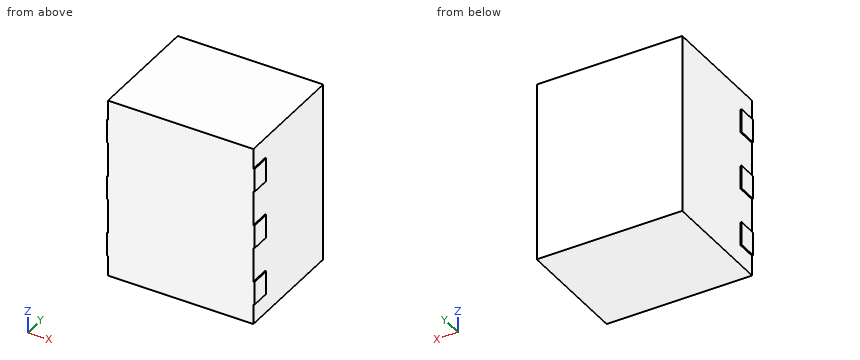
Autodesk Inventor part; units mm, degrees
ref_plane "YZ Plane" through (0, 0, 0) normal (1, 0, 0) x (0, 1, 0)
ref_plane "XZ Plane" through (0, 0, 0) normal (0, 1, 0) x (-1, 0, 0)
ref_plane "XY Plane" through (0, 0, 0) normal (0, 0, 1) x (1, 0, 0)
sketch "Sketch1" plane through (0, 0, 0) normal (0, 1, 0) x (-1, 0, 0)
  line L0 (3.175, 3.935) -> (-3.175, 3.935)
  line L1 (-3.175, 3.935) -> (-3.175, -3.935)
  line L2 (-3.175, -3.935) -> (3.175, -3.935)
  line L3 (3.175, -3.935) -> (3.175, 3.935)
  point P0 (0, 0)
  dimension "d0" = 6.35
  dimension "d1" = 3.175
  dimension "d2" = 7.87
  dimension "d3" = 3.935
extrude "Extrusion1" add sketch "Sketch1" along normal blind 5.08
sketch "Sketch2" plane through (0, 0, 0) normal (0, -1, 0) x (1, 0, 0)
  line L0 (3.225, 0.51) -> (1.955, 0.51)
  line L1 (1.955, 0.51) -> (1.955, -0.51)
  line L2 (1.955, -0.51) -> (3.225, -0.51)
  line L3 (3.225, -0.51) -> (3.225, 0.51)
  line L4 (3.175, 3.935) -> (3.175, -3.935)
  point P0 (0, 0)
  dimension "d6" = 1.02
  dimension "d7" = 0.51
  dimension "d8" = 0.05
  dimension "d9" = 1.27
extrude "Extrusion2" add sketch "Sketch2" against normal blind 0.8467
pattern_linear "Rectangular Pattern1" count 3 spacing 2.54 along (0, 0, -1) of "Extrusion2" first direction both ways yes
mirror "Mirror1" about plane through (0, 0, 0) normal (1, 0, 0) of "Extrusion2", "Rectangular Pattern1"
properties part number "MC_TT240"
The model under review builds one solid part; all positions refer to its coordinate system, in mm. Coordinates: 2 decimals unless noted, no trailing zeros. Order: outer loops, then holes, each group sorted by start corner. A loop starts at its lowest first (then second) coordinate and runs counter-clockwise, first axis right, second up. Notation, with made-up numbers: (-9.75, -22.5) -> (25.25, -22.5) arc R24 cw to (25.25, 0.5) -> close; hole circle Ø8 at (28, 75). An arc over 180 degrees is marked (long way). Answer in a Markdown table with one row per item. Add a question column.
Item 1: Clearance check with a flat-ended pin moving along its axis: pin 1 (1 mm diameter, centred on y = 4.5, z = 3, fed in from -X) (3 decimals). State where the tip first meets the part, or that it passes through.
Item 2: We need section A-A on y = 2.6. Write out the cut boundary in (x, z) (3 decimals).
Item 3: To check wall thickness, follow probe 1 along X at (y, z) = (4.85, -1.5) (3 decimals). State the ranges of the line that lie inside material, in increasing order.
Item 4: We need section B-B on z = 1.5. Write out the cut boundary in (x, y) (3 decimals), plus the area to 3 significant figures.
Final values:
| question | item | result |
|---|---|---|
| 1 | pin 1 | stops at x = -3.175 |
| 2 | outline | (-3.175, -3.935) -> (3.175, -3.935) -> (3.175, 3.935) -> (-3.175, 3.935) -> close |
| 3 | probe 1 | x = -3.175 to 3.175 |
| 4 | outline | (-3.175, 0) -> (3.175, 0) -> (3.175, 5.08) -> (-3.175, 5.08) -> close |
| 4 | area | 32.3 mm2 |
